```python
from build123d import *

# Parameters (mm, degrees)
F0_W      = 358.775
F0_H      = 698.5
F1_DEPTH  = 581.025
F2_W      = 333.375
F2_H      = 673.1
F2_W_2    = 330.835
F2_H_2    = 670.56
F3_DEPTH  = 304.8
F4_W      = 330.835
F4_H      = 1.27
F4_W_2    = 333.375
F4_W_3    = 332.105
F5_DEPTH  = 304.8
F7_DEPTH  = 304.8
F8_R      = 50.8
F10_DEPTH = 304.8
F11_R     = 50.8
F13_DEPTH = 304.8
F14_R     = 50.8
F16_DEPTH = 304.8
F17_R     = 50.8
F19_DEPTH = 304.8
F20_R     = 50.8


with BuildPart() as f1:
    # F0 (on Front) → F1 (new body)
    with BuildSketch(Plane.XZ):
        with Locations((130.6179589152, 307.5007573068)):
            Rectangle(F0_W, F0_H)
    extrude(amount=F1_DEPTH)

    # F2 (on face) → F3 (cut)
    with BuildSketch(Plane.XZ.offset(581.025)):
        with Locations((130.6179589152, 307.5007573068)):
            Rectangle(F2_W, F2_H)
        with Locations((130.6179589152, 307.5007573068)):
            Rectangle(F2_W_2, F2_H_2, mode=Mode.SUBTRACT)
    extrude(amount=-F3_DEPTH, mode=Mode.SUBTRACT)

    # F4 (on face) → F5 (cut)
    with BuildSketch(Plane.XZ.offset(581.025)):
        with Locations((130.6179589152, 556.4207573068)):
            Rectangle(F4_W, F4_H)
        with Locations((130.6179589152, 469.4257573068)):
            Rectangle(F4_W_2, F4_H)
        with Locations((129.9829589152, 303.5637573068)):
            Rectangle(F4_W_3, F4_H)
        with Locations((131.2529589152, 137.7017573068)):
            Rectangle(F4_W_3, F4_H)
    extrude(amount=-F5_DEPTH, mode=Mode.SUBTRACT)

    # F6 (on face) → F7 (cut)
    with BuildSketch(Plane.XZ.offset(581.025)):
        Polygon((218.0892089152, 642.7807573068), (43.1467089152, 642.7807573068), (81.2467089152, 630.0807573068), (179.9892089152, 630.0807573068), align=None)
    extrude(amount=-F7_DEPTH, mode=Mode.SUBTRACT)

    # F8
    f8_edges = [f1.edges().sort_by_distance(p)[0] for p in [
        (43.146709, -428.625, 642.780757),
        (81.246709, -428.625, 630.080757),
        (179.989209, -428.625, 630.080757),
        (218.089209, -428.625, 642.780757),
    ]]
    fillet(f8_edges, radius=F8_R)

    # F9 (on face) → F10 (cut)
    with BuildSketch(Plane.XZ.offset(581.025)):
        Polygon((218.0892089152, 555.7857573068), (43.1467089152, 555.7857573068), (81.2467089152, 543.0857573068), (179.9892089152, 543.0857573068), align=None)
    extrude(amount=-F10_DEPTH, mode=Mode.SUBTRACT)

    # F11
    f11_edges = [f1.edges().sort_by_distance(p)[0] for p in [
        (43.146709, -428.625, 555.785757),
        (81.246709, -428.625, 543.085757),
        (218.089209, -428.625, 555.785757),
        (179.989209, -428.625, 543.085757),
    ]]
    fillet(f11_edges, radius=F11_R)

    # F12 (on face) → F13 (cut)
    with BuildSketch(Plane.XZ.offset(581.025)):
        Polygon((218.0892089152, 468.7907573068), (43.1467089152, 468.7907573068), (81.2467089152, 456.0907573068), (179.9892089152, 456.0907573068), align=None)
    extrude(amount=-F13_DEPTH, mode=Mode.SUBTRACT)

    # F14
    f14_edges = [f1.edges().sort_by_distance(p)[0] for p in [
        (43.146709, -428.625, 468.790757),
        (81.246709, -428.625, 456.090757),
        (179.989209, -428.625, 456.090757),
        (218.089209, -428.625, 468.790757),
    ]]
    fillet(f14_edges, radius=F14_R)

    # F15 (on face) → F16 (cut)
    with BuildSketch(Plane.XZ.offset(581.025)):
        Polygon((218.0892089152, 302.9287573068), (43.1467089152, 302.9287573068), (81.2467089152, 290.2287573068), (179.9892089152, 290.2287573068), align=None)
    extrude(amount=-F16_DEPTH, mode=Mode.SUBTRACT)

    # F17
    f17_edges = [f1.edges().sort_by_distance(p)[0] for p in [
        (43.146709, -428.625, 302.928757),
        (81.246709, -428.625, 290.228757),
        (179.989209, -428.625, 290.228757),
        (218.089209, -428.625, 302.928757),
    ]]
    fillet(f17_edges, radius=F17_R)

    # F18 (on face) → F19 (cut)
    with BuildSketch(Plane.XZ.offset(581.025)):
        Polygon((218.0892089152, 137.0667573068), (43.1467089152, 137.0667573068), (81.2467089152, 124.3667573068), (179.9892089152, 124.3667573068), align=None)
    extrude(amount=-F19_DEPTH, mode=Mode.SUBTRACT)

    # F20
    f20_edges = [f1.edges().sort_by_distance(p)[0] for p in [
        (43.146709, -428.625, 137.066757),
        (81.246709, -428.625, 124.366757),
        (179.989209, -428.625, 124.366757),
        (218.089209, -428.625, 137.066757),
    ]]
    fillet(f20_edges, radius=F20_R)


solid = f1.part
```
Read the model definition and answer for the solid it produces. Units are mm, in the model's axes. A direction names the side the tool comes from. Round coordinates to 2 decimals unless told otherwise and drop trailing zeros. Write each loop counter-clockwise with the first axis right and the second up, starting at its lowest first coordinate (ties: lowest second). Pieces come first, ordered by that corner, then holes. Notation, with made-up numbers: (24, -39.5) -> (36, -39.5) arc R25 ccw to (36, -7.5) -> close; hole circle Ø8 at (43.25, 71.25). An arc over 180 degrees is marked (long way). Answer in a Markdown table with one row per item. Add a question column.
1) Determine the mould class of faces 1 (the face through (-43, -581.025, 413)), 2 (the face through (128, -286, 656.751)), 3 (the face through (261, -431, 555.786)) for opening direction Z: pulls with the +Z half, pulls with the -Z half, needs draft (parallel to the pull), parting line crosses it, or undercut.
2) Which of the six approach directions +Z, -Z, +X, -X, +Y, -Y give full straight-line access (tool end or side, diameter ignored) to faces 4 (the face through (128, -581.025, 388)), 5 (the face through (81.24, -426.49, 125.04))?
3) Find section B-B, the plane x = 162. Determine the outline of the cut face in (y, z) (3 decimals).
4) Find section A-A, the plane y = -304.5. State how many separate pieces and enclosed holes the cut face has, and give its area (3 significant figures).
5) Consider line 1 (X direction, y = -434, z = -3); line 2 (Y direction, x = 111, z = 299) (3 decimals). Determine where each line is inside the solid, lowest interval first.
Findings below:
| question | item | result |
|---|---|---|
| 1 | face 1 | needs draft |
| 1 | face 2 | pulls with the +Z half |
| 1 | face 3 | undercut |
| 2 | face 4 | +Z, -Z, +X, -X, -Y |
| 2 | face 5 | -Y |
| 3 | outline | (-581.025, -41.749) -> (0, -41.749) -> (0, 656.751) -> (-581.025, 656.751) -> (-581.025, 644.051) -> (-276.225, 644.051) -> (-276.225, 630.081) -> (-581.025, 630.081) -> (-581.025, 557.056) -> (-276.225, 557.056) -> (-276.225, 543.086) -> (-581.025, 543.086) -> (-581.025, 470.061) -> (-276.225, 470.061) -> (-276.225, 456.091) -> (-581.025, 456.091) -> (-581.025, 304.199) -> (-276.225, 304.199) -> (-276.225, 290.229) -> (-581.025, 290.229) -> (-581.025, 138.337) -> (-276.225, 138.337) -> (-276.225, 124.367) -> (-581.025, 124.367) -> (-581.025, -27.779) -> (-276.225, -27.779) -> (-276.225, -29.049) -> (-581.025, -29.049) -> close |
| 4 | separate pieces | 6 |
| 4 | enclosed holes | 1 |
| 4 | area | 238,000 mm² |
| 5 | line 1 | -48.77 to -36.07, -34.8 to 296.04, 297.31 to 310.01 |
| 5 | line 2 | -276.225 to 0 |
